Can you work these out from the model? Positions are in its coordinate system, mm. Face numbers are marked on the shaded views. A direction names the side the tool comes from. Round coordinates to 2 decimals unless told otherwise and drop trailing zeros. Order: outer loops, then holes, each group sorted by start corner. A loop starts at its lowest first (then second) coordinate and runs counter-clockwise, first axis right, second up.
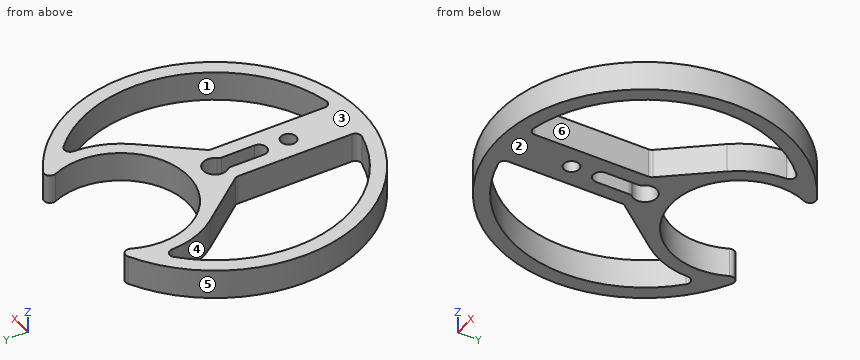
Autodesk Inventor part; units mm, degrees
ref_plane "YZ Plane" through (0, 0, 0) normal (1, 0, 0) x (0, 1, 0)
ref_plane "XZ Plane" through (0, 0, 0) normal (0, 1, 0) x (-1, 0, 0)
ref_plane "XY Plane" through (0, 0, 0) normal (0, 0, 1) x (1, 0, 0)
sketch "Sketch1" plane through (0, 0, 0) normal (0, 0, 1) x (1, 0, 0)
  circle A0 centre (0, 0) radius 60.5521
  arc A1 (-0.7258, 10.3355) -> (0.2666, 10.325) centre (0, 32) ccw
  circle A2 centre (0, 0) radius 60.5521
  circle A3 centre (0, 32) radius 2.5
  circle A4 centre (0, 0) radius 50
  circle A5 centre (0, 0) radius 57.5
  circle A6 centre (0, 0) radius 57
  circle A7 centre (0, 0) radius 7.5
  circle A8 centre (0, 32) radius 23
  circle A9 centre (0, 0) radius 45
  circle A10 centre (0, 32) radius 27.5
  line L0 (-5.8547, -4.6875) -> (-21.4672, 14.8125)
  line L1 (5.8547, -4.6875) -> (21.4672, 14.8125)
  line L2 (0, 0) -> (0, 32)
  line L3 (7.5, 44.3706) -> (7.5, -44.3706)
  line L4 (-7.5, 44.3706) -> (-7.5, -44.3706)
  circle A11 centre (0, 0) radius 2.6
  line L5 (0, 0) -> (0, -15)
  circle A12 centre (0, -15) radius 2.6
  line L6 (-2.6, -15) -> (-2.6, 0)
  line L7 (2.6, 0) -> (2.6, -15)
  circle A13 centre (0, 0) radius 4
  line L8 (0, -15) -> (0, -25)
  circle A14 centre (0, -25) radius 2.6
  point P0 (27.2328, 35.8242)
  point P1 (7.5, -2.6325)
  point P2 (-27.2328, 35.8242)
  point P3 (-7.5, -2.6325)
  point P4 (17.6083, 46.7969)
  point P5 (-17.6083, 46.7969)
  point P6 (-2.6, -3.0397)
  point P7 (2.6, -3.0397)
  dimension "d0" = 5
  dimension "d1" = 100
  dimension "d2" = 115
  dimension "d4" = 15
  dimension "d5" = 46
  dimension "d6" = 90
  dimension "d7" = 55
  dimension "d8" = 32
  dimension "d12" = 5.2
  dimension "d13" = 15
  dimension "d14" = 5.2
  dimension "d15" = 8
  dimension "d17" = 10
  dimension "d18" = 5.2
extrude "Extrusion1" add sketch "Sketch1" along normal blind 10 contours A8 L3 A10 A7 L2 | L2 A7 A10 L4 A8 | L4 A10 A9 A8 | A8 A9 A10 L3 | L2 A10 A7 | A7 A10 L2 | A9 A10 A4 A8 | L4 L0 A10 | A10 A7 L4 | L3 A7 A10 | A10 L1 L3 | A7 L7 A13 L2 A10 | A10 L2 A13 L6 A7 | A9 A10 A4 | A7 L0 L4 | A8 A4 A10 A9 | L3 L1 A7 | L4 L0 A7 L6 A12 L7 L1 L3 A9
fillet "Fillet1" radius 2 8 edges at (-17.6083, 46.7969, 5) (17.6083, 46.7969, 5) (27.2328, 35.8242, 5) (-27.2328, 35.8242, 5) (-7.5, -2.6325, 5) (7.5, -2.6325, 5) (7.5, -44.3706, 5) (-7.5, -44.3706, 5)
fillet "Fillet2" radius 2 2 edges at (-2.6, -3.0397, 5) (2.6, -3.0397, 5)
properties part number "Gear Holder 1"
(1) If we mould it in two halves opening along X, with no side actions, what happens to the marked faces 3, 4, 5 and 6? For each: pulls with the +X half, pulls with the -X half, needs draft (parallel to the pull), parting line crosses it, or undercut.
(2) I want a section at A-A, the plane y = 17. List the corners of the cut face in (x, z) for me.
(3) I'm going to push flat-ended pins straight in: pin 1 Ø5 at (x, z) = (-29.5, 3.5) entering from -Y; pin 2 Ø3 at (y, z) = (-12, 3) entering from +X; pin 3 Ø2 at (y, z) = (14.5, 2.5) entering from +X. Where does each tip first touch, or does it pass through?
(4) On a 3-axis mill with a long thin cutter (end or side, diameter ignored), from which of +Z, -Z, +X, -X, +Y, -Y can I reach the whole of each face in a straight line? I mean the marked faces 1 and 2. Say none if no direction works.
(5) I want a section at B-B, the plane x = 0. List the corners of the cut face in (y, z) for me, plus the area to 3 significant figures.
(6) I want a section at C-C, the plane x = 13. List the corners of the cut face in (y, z) for me, plus the area to 3 significant figures.
(7) Please list where these lines run through material, in increasing order: probe 1 along Y at (x, z) = (0, 5.25); probe 2 along X at (y, z) = (-21, 6.5); probe 3 along X at (y, z) = (19, 6).
(8) I want a section at D-D, the plane y = 0. List the corners of the cut face in (x, z) for me, plus the area to 3 significant figures.
Ans:
1. face 3: needs draft
1. face 4: undercut
1. face 5: parting line crosses it
1. face 6: undercut
2. outline: (-47.02, 0) - (-41.67, 0) - (-41.67, 10) - (-47.02, 10) - close; (-23.05, 0) - (-17.44, 0) - (-17.44, 10) - (-23.05, 10) - close; (17.44, 0) - (23.05, 0) - (23.05, 10) - (17.44, 10) - close; (41.67, 0) - (47.02, 0) - (47.02, 10) - (41.67, 10) - close
3. pin 1: stops at y = -42.08
3. pin 2: stops at x = 48.89
3. pin 3: stops at x = 48.14
4. face 1: +Z, -Z
4. face 2: -Z, +X, -X, +Y, -Y
5. outline: (-50, 0) - (-27.6, 0) - (-27.6, 10) - (-50, 10) - close; (-22.4, 0) - (-17.6, 0) - (-17.6, 10) - (-22.4, 10) - close; (4, 0) - (9, 0) - (9, 10) - (4, 10) - close
5. area: 322 mm2
6. outline: (-48.28, 0) - (-43.08, 0) - (-43.08, 10) - (-48.28, 10) - close; (4.24, 0) - (13.03, 0) - (13.03, 10) - (4.24, 10) - close
6. area: 140 mm2
7. probe 1: y = -50 to -27.6, -22.4 to -17.6, 4 to 9
7. probe 2: x = -45.38 to -39.8, -7.5 to 7.5, 39.8 to 45.38
7. probe 3: x = -46.25 to -40.79, -24.23 to -18.97, 18.97 to 24.23, 40.79 to 46.25
8. outline: (-50, 0) - (-45, 0) - (-45, 10) - (-50, 10) - close; (-9.61, 0) - (-4, 0) - (-4, 10) - (-9.61, 10) - close; (4, 0) - (9.61, 0) - (9.61, 10) - (4, 10) - close; (45, 0) - (50, 0) - (50, 10) - (45, 10) - close
8. area: 212 mm2
